Input: part model. Units: mm. Frame: model coordinates. A direction names the side the tool comes from. Round coordinates to 2 decimals unless told otherwise and drop trailing zeros. Loops run counter-clockwise (first coordinate to the right, second up) from the corner with the lowest first, then second, coordinate; pieces in that order, holes last. Notation, with made-up numbers: (2.5, -3) - (51.5, -3) arc R20 cw to (51.5, 28) - close; hole circle Ø2 at (-14, 82). An arc over 180 degrees is marked (long way). One line per question, with ' | ' between items. Start each with the question number.
Item 1: Section C-C, the plane y = -13. Return loops of the section in (x, z), plus the area to 3 significant figures.
Item 2: Section D-D, the plane z = 2.75. Return loops of the section in (x, y).
Item 3: Draft query along Y for faces 4 (the face through (-2.956, -9.974, 0.014)), 5 (the face through (11.72, -6.69, 0.01)), 6 (the face through (-3.045, 10.041, 0.014)). Return one class per face: pulls with the +Y half, pulls with the -Y half, needs draft (parallel to the pull), parting line crosses it, or undercut.
Item 4: Section A-A, the plane y = -8. Return loops of the section in (x, z), plus the area to 3 significant figures.
Item 5: Material intervals for line 1 along Y through (x, z) = (0, 0.1); line 2 along Y through (x, z) = (0, 2.8); line 3 along Y through (x, z) = (11, -0.6), sorted ascending.
Item 6: Section B-B, the plane z = -0.2. Return loops of the section in (x, y).
Item 7: First-contact query: pin 1 (5 mm diameter, centred on x = 0, y = 0, fed in from -Z); pin 2 (2 mm diameter, centred on x = 0.5, y = -1, fed in from +Z); pin 3 (1.5 mm diameter, centred on y = 3, z = -0.5, fed in from +X); pin 4 (1.5 mm diameter, centred on x = -1.5, z = 2, fed in from -Y). Flat tips, straight axial feed; report the tip coordinate or a pass-through.
Item 8: Set-up query: faces 1 (the face through (10.218, -2.383, 0.014)), 2 (the face through (-7.159, 7.547, 0.014)), 3 (the face through (-10.12, -2.43, 0.01)). Return all of +Z, -Z, +X, -X, +Y, -Y with unobstructed straight access to the full face (end or side cutting, diameter ignored); none if empty.
```python
from build123d import *

# Parameters (mm, degrees)
ESBO_O1_R                = 1.5
RESSALTO_EXTRUS_O1_DEPTH = 1
ESBO_O2_R                = 4.25
ESBO_O2_R_2              = 3.25
RESSALTO_EXTRUS_O2_DEPTH = 3
ESBO_O3_R                = 0.5
CORTE_EXTRUS_O1_DEPTH    = 2


with BuildPart() as part:
    # Esboço1 → Ressalto-extrusão1 (new body, symmetric)
    with BuildSketch(Plane.XY):
        with BuildLine():
            Line((3.75, 6.495190528), (2.140193877, 13.55121581))
            ThreePointArc((2.140193877, 13.55121581), (-0.135352736, 15.340099778), (-2.359806123, 13.488067011))
            Line((-2.359806123, 13.488067011), (-3.75, 6.495190528))
            Line((-3.75, 6.495190528), (-10.665600205, 8.629070172))
            ThreePointArc((-10.665600205, 8.629070172), (-13.352592472, 7.552830981), (-12.86091174, 4.700381455))
            Line((-12.86091174, 4.700381455), (-7.5, 0))
            Line((-7.5, 0), (-12.805794082, -4.922145638))
            ThreePointArc((-12.805794082, -4.922145638), (-13.217239736, -7.787268797), (-10.501105618, -8.787685556))
            Line((-10.501105618, -8.787685556), (-3.75, -6.495190528))
            Line((-3.75, -6.495190528), (-2.140193877, -13.55121581))
            ThreePointArc((-2.140193877, -13.55121581), (0.135352736, -15.340099778), (2.359806123, -13.488067011))
            Line((2.359806123, -13.488067011), (3.75, -6.495190528))
            Line((3.75, -6.495190528), (10.665600205, -8.629070172))
            ThreePointArc((10.665600205, -8.629070172), (13.352592472, -7.552830981), (12.86091174, -4.700381455))
            Line((12.86091174, -4.700381455), (7.5, 0))
            Line((7.5, 0), (12.805794082, 4.922145638))
            ThreePointArc((12.805794082, 4.922145638), (13.217239736, 7.787268797), (10.501105618, 8.787685556))
            Line((10.501105618, 8.787685556), (3.75, 6.495190528))
        make_face()
        Circle(ESBO_O1_R, mode=Mode.SUBTRACT)
    extrude(amount=RESSALTO_EXTRUS_O1_DEPTH, both=True)

    # Esboço2 → Ressalto-extrusão2 (add)
    with BuildSketch(Plane.XY.offset(1)):
        Circle(ESBO_O2_R)
        Circle(ESBO_O2_R_2, mode=Mode.SUBTRACT)
    extrude(amount=RESSALTO_EXTRUS_O2_DEPTH)

    # Esboço3 → Corte-extrusão1 (cut)
    with BuildSketch(Plane.XY.offset(1)):
        with Locations((0, 13)):
            Circle(ESBO_O3_R)
        with Locations((11.258330249, 6.5)):
            Circle(ESBO_O3_R)
        with Locations((11.258330249, -6.5)):
            Circle(ESBO_O3_R)
        with Locations((0, -13)):
            Circle(ESBO_O3_R)
        with Locations((-11.258330249, -6.5)):
            Circle(ESBO_O3_R)
        with Locations((-11.258330249, 6.5)):
            Circle(ESBO_O3_R)
    extrude(amount=-CORTE_EXTRUS_O1_DEPTH, mode=Mode.SUBTRACT)


solid = part.part
```
Return value:
1) outline: (-2.27, -1) - (-0.5, -1) - (-0.5, 1) - (-2.27, 1) - close; (0.5, -1) - (2.46, -1) - (2.46, 1) - (0.5, 1) - close | area: 7.45 mm2
2) outline: circle Ø8.5 at (0, 0); hole circle Ø6.5 at (0, 0)
3) face 4: pulls with the -Y half | face 5: undercut | face 6: pulls with the +Y half
4) outline: (-13.07, -1) - (-8.18, -1) - (-8.18, 1) - (-13.07, 1) - close; (-3.41, -1) - (3.45, -1) - (3.45, 1) - (-3.41, 1) - close; (8.63, -1) - (13.03, -1) - (13.03, 1) - (8.63, 1) - close | area: 32.3 mm2
5) line 1: -15.34 to -13.5, -12.5 to -1.5, 1.5 to 12.5, 13.5 to 15.34 | line 2: -4.25 to -3.25, 3.25 to 4.25 | line 3: -8.71 to -6.93, -6.07 to -3.07, 3.25 to 6.07, 6.93 to 8.9
6) outline: (-12.86, 4.7) - (-7.5, 0) - (-12.81, -4.92) arc R2.3 ccw to (-10.5, -8.79) - (-3.75, -6.5) - (-2.14, -13.55) arc R2.3 ccw to (2.36, -13.49) - (3.75, -6.5) - (10.67, -8.63) arc R2.3 ccw to (12.86, -4.7) - (7.5, 0) - (12.81, 4.92) arc R2.3 ccw to (10.5, 8.79) - (3.75, 6.5) - (2.14, 13.55) arc R2.3 ccw to (-2.36, 13.49) - (-3.75, 6.5) - (-10.67, 8.63) arc R2.3 ccw to start; hole circle Ø1 at (-11.26, -6.5); hole circle Ø1 at (-11.26, 6.5); hole circle Ø3 at (0, 0); hole circle Ø1 at (0, -13); hole circle Ø1 at (0, 13); hole circle Ø1 at (11.26, -6.5); hole circle Ø1 at (11.26, 6.5)
7) pin 1: z = -1 | pin 2: z = 1 | pin 3: x = 11.54 | pin 4: y = -4.18
8) face 1: +Z, -Z, +X | face 2: +Z, -Z, +Y | face 3: +Z, -Z, -X
